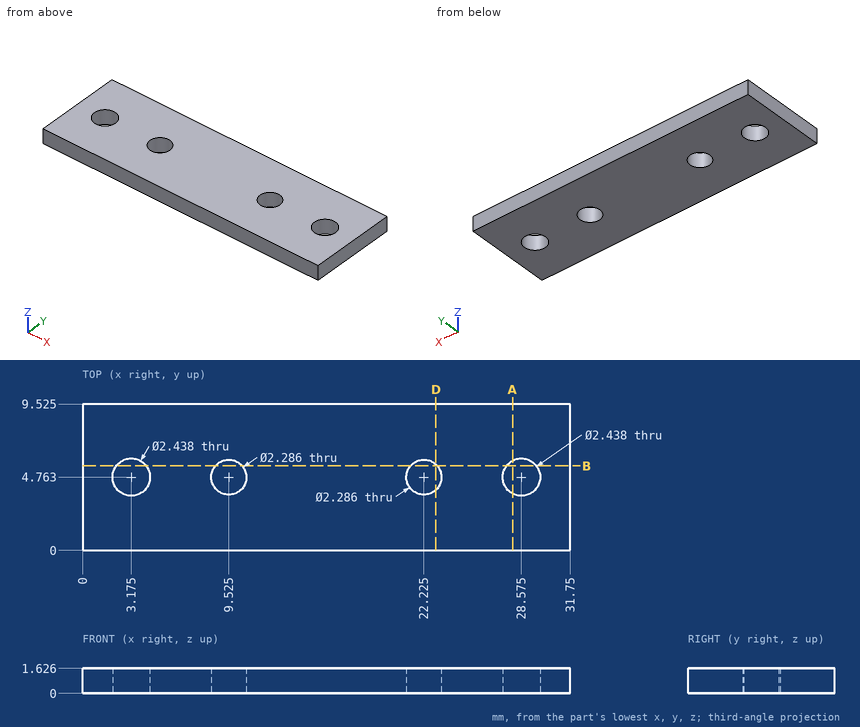
Part print with two shaded views. Sizes in mm from the minimum x, y, z corner. Round coordinates to 2 decimals unless told otherwise and drop trailing zeros. Loops run counter-clockwise (first coordinate to the right, second up) from the corner with the lowest first, then second, coordinate; pieces in that order, holes last. Notation, with made-up numbers: M 13.25,79 L 70.25,79 A26 cw 70.25,99 Z; hole C 1,8 d5. An arc over 180 degrees is marked long. Return JSON: item names as keys, results as strings. Group by question number.
(1) Saw through at B-B, the plane y = 5.5. Give the number of separate pieces and of enclosed holes in the cut face.
(2) Saw through at D-D, the plane x = 23. List the corners of the cut face in (y, z) (1 decimal).
(3) Saw through at A-A, the plane x = 28. List the corners of the cut face in (y, z) (1 decimal), and give its area (3 significant figures).
(4) Drop a flat-ended pin along its axis: P1, Ø2, axis at x = 9.52, y = 4.76, coming from the -Z side. Give the stop position or say it passes through.
(5) Wall check: probe 1 along Y at (x, z) = (10, 1.15) (1 decimal); probe 2 along Y at (x, z) = (29, 0.4) (1 decimal). Give the ranges that are in metal, low to high. Write a range as [from, to].
Answer list:
{
 "1": {"separate pieces": "5", "enclosed holes": "0"},
 "2": {"outline": "M 0,0 L 3.9,0 L 3.9,1.6 L 0,1.6 Z; M 5.6,0 L 9.5,0 L 9.5,1.6 L 5.6,1.6 Z"},
 "3": {"outline": "M 0,0 L 3.7,0 L 3.7,1.6 L 0,1.6 Z; M 5.8,0 L 9.5,0 L 9.5,1.6 L 5.8,1.6 Z", "area": "12.0 mm2"},
 "4": {"P1": "through"},
 "5": {"probe 1": "[0, 3.7], [5.8, 9.5]", "probe 2": "[0, 3.6], [5.9, 9.5]"}
}
